Can you work these out from the model? Positions are in its coordinate system, mm. Face numbers are marked on the shaded views. A direction names the side the tool comes from. Give positions to 0.01 mm unless a question says otherwise; leave off trailing zeros. Loops run counter-clockwise (first coordinate to the right, second up) from the corner with the lowest first, then second, coordinate; pieces in that order, holes last.
Autodesk Fusion 360 part; units mm, degrees
sketch "Sketch1" plane through (0, 0, 0) normal (0, 0, 1) x (1, 0, 0)
  line L0 (10, 0) -> (59, 0)
  line L1 (69, 10) -> (69, 170)
  line L2 (59, 180) -> (10, 180)
  line L3 (0, 170) -> (0, 10)
  arc A0 (10, 180) -> (0, 170) centre (10, 170) ccw
  arc A1 (69, 170) -> (59, 180) centre (59, 170) ccw
  arc A2 (59, 0) -> (69, 10) centre (59, 10) ccw
  arc A3 (0, 10) -> (10, 0) centre (10, 10) ccw
  point P0 (69, 0)
  point P1 (0, 180)
  dimension "d1" = 69
  dimension "d2" = 180
  dimension "d3" = 10
  dimension "d4" = 10
  dimension "d5" = 10
sketch "Sketch2" plane through (0, 0, 27) normal (0, 0, 1) x (-1, 0, 0)
  line L0 (-10, 0) -> (-59, 0)
  arc A0 (-59, 0) -> (-69, -10) centre (-59, -10) ccw
sketch "Sketch3" plane through (0, 0, 0) normal (0, 0, 1) x (1, 0, 0)
  line L0 (15, 0) -> (54, 0)
  line L1 (69, 15) -> (69, 180)
  line L2 (54, 195) -> (15, 195)
  line L3 (0, 180) -> (0, 15)
  circle A0 centre (34.5, 110) radius 11
  circle A1 centre (34.5, 85) radius 11
  circle A2 centre (34.5, 128.9) radius 5
  circle A3 centre (34.5, 66.1) radius 5
  circle A4 centre (34.5, 47.2) radius 11
  circle A5 centre (34.5947, 147.7998) radius 11
  circle A6 centre (34.5, 22.2) radius 11
  circle A7 centre (34.4989, 172.7996) radius 11
  arc A8 (15, 195) -> (0, 180) centre (15, 180) ccw
  arc A9 (69, 180) -> (54, 195) centre (54, 180) ccw
  arc A10 (54, 0) -> (69, 15) centre (54, 15) ccw
  arc A11 (0, 15) -> (15, 0) centre (15, 15) ccw
  circle A12 centre (54, 160.2997) radius 4
  point P0 (69, 0)
  dimension "d76" = 22
  dimension "d77" = 22
  dimension "d78" = 18.9
  dimension "d79" = 18.9
  dimension "d80" = 10
  dimension "d81" = 10
  dimension "d82" = 18.9
  dimension "d83" = 18.9
  dimension "d84" = 22
  dimension "d85" = 22
  dimension "d86" = 25
  dimension "d87" = 25
  dimension "d88" = 22
  dimension "d89" = 22
  dimension "d90" = 15
  dimension "d91" = 15
  dimension "d92" = 15
  dimension "d93" = 15
  dimension "d130" = 8
sketch "Sketch4" plane through (0, 0, 27) normal (0, 0, 1) x (-1, 0, 0)
sketch "Sketch5" plane through (0, 0, 0) normal (0, 0, 1) x (1, 0, 0)
extrude "Extrude2" add sketch "Sketch3" along normal blind 27
sketch "Sketch6" plane through (0, 0, 0) normal (0, 0, -1) x (1, 0, 0)
  circle A0 centre (54, -160.2997) radius 4
  circle A1 centre (34.4989, -172.7996) radius 11
  circle A2 centre (34.5, -110) radius 11
  circle A3 centre (34.5947, -147.7998) radius 11
  circle A4 centre (34.5, -85) radius 11
  circle A5 centre (34.5, -66.1) radius 5
  circle A6 centre (34.5, -47.2) radius 11
  circle A7 centre (34.5, -22.2) radius 11
  circle A8 centre (34.5, -128.9) radius 5
  arc A9 (15, 0) -> (0, -15) centre (15, -15) ccw
  line L0 (0, -15) -> (0, -180)
  arc A10 (0, -180) -> (15, -195) centre (15, -180) ccw
  line L1 (15, -195) -> (54, -195)
  arc A11 (54, -195) -> (69, -180) centre (54, -180) ccw
  line L2 (69, -180) -> (69, -15)
  arc A12 (69, -15) -> (54, 0) centre (54, -15) ccw
  line L3 (54, 0) -> (15, 0)
  line L4 (34.5, -85) -> (0, -85)
  line L5 (15, -5) -> (54, -5)
  line L6 (64, -15) -> (64, -180)
  line L7 (54, -190) -> (15, -190)
  line L8 (5, -180) -> (5, -15)
  arc A13 (15, -5) -> (5, -15) centre (15, -15) ccw
  arc A14 (64, -15) -> (54, -5) centre (54, -15) ccw
  arc A15 (5, -180) -> (15, -190) centre (15, -180) ccw
  arc A16 (54, -190) -> (64, -180) centre (54, -180) ccw
  dimension "d162" = 10
  dimension "d163" = 10
  dimension "d164" = 10
  dimension "d165" = 10
extrude "Extrude3" cut sketch "Sketch6" against normal blind 22 contours L5 L6 L7 L8 A13 A14 A15 A16
sketch "Sketch7" plane through (0, 0, 27) normal (0, 0, 1) x (-1, 0, 0)
  circle A0 centre (-54, -160.2997) radius 4
  circle A1 centre (-34.4989, -172.7996) radius 11
  circle A2 centre (-34.5, -110) radius 11
  circle A3 centre (-34.5947, -147.7998) radius 11
  circle A4 centre (-34.5, -85) radius 11
  circle A5 centre (-34.5, -66.1) radius 5
  circle A6 centre (-34.5, -47.2) radius 11
  circle A7 centre (-34.5, -22.2) radius 11
  circle A8 centre (-34.5, -128.9) radius 5
  arc A9 (0, -15) -> (-15, 0) centre (-15, -15) ccw
  line L0 (-15, 0) -> (-54, 0)
  arc A10 (-54, 0) -> (-69, -15) centre (-54, -15) ccw
  line L1 (-69, -15) -> (-69, -180)
  arc A11 (-69, -180) -> (-54, -195) centre (-54, -180) ccw
  line L2 (-54, -195) -> (-15, -195)
  arc A12 (-15, -195) -> (0, -180) centre (-15, -180) ccw
  line L3 (0, -180) -> (0, -15)
sketch "Sketch8" plane through (0, 0, 0) normal (0, 0, -1) x (1, 0, 0)
  line L0 (54, -190) -> (15, -190)
  arc A0 (5, -180) -> (15, -190) centre (15, -180) ccw
  line L1 (5, -180) -> (5, -15)
  arc A1 (15, -5) -> (5, -15) centre (15, -15) ccw
  line L2 (15, -5) -> (54, -5)
  arc A2 (64, -15) -> (54, -5) centre (54, -15) ccw
  line L3 (64, -15) -> (64, -180)
  arc A3 (54, -190) -> (64, -180) centre (54, -180) ccw
  arc A4 (15, 0) -> (0, -15) centre (15, -15) ccw
  line L4 (0, -15) -> (0, -180)
  arc A5 (0, -180) -> (15, -195) centre (15, -180) ccw
  line L5 (15, -195) -> (54, -195)
  arc A6 (54, -195) -> (69, -180) centre (54, -180) ccw
  line L6 (69, -180) -> (69, -15)
  arc A7 (69, -15) -> (54, 0) centre (54, -15) ccw
  line L7 (54, 0) -> (15, 0)
  line L8 (0, -34.7) -> (0, -29.7)
  line L9 (0, -34.7) -> (0, -39.7)
  line L10 (0, -39.7) -> (0, -29.7)
  line L11 (0, -29.7) -> (5, -29.7)
  line L12 (0, -39.7) -> (5, -39.7)
  line L13 (5, -29.7) -> (5, -39.7)
extrude "Extrude4" cut sketch "Sketch8" against normal blind 5 contours L1 L4 L8 L9 L10 L11 L12 L13
sketch "Sketch9" plane through (0, 0, 0) normal (-1, 0, 0) x (0, -1, 0)
  line L0 (-39.7, 0) -> (-39.7, 5)
  line L1 (-39.7, 5) -> (-29.7, 5)
  line L2 (-29.7, 5) -> (-29.7, 0)
  line L3 (-29.7, 0) -> (-15, 0)
  line L4 (-15, 0) -> (-15, 27)
  line L5 (-15, 27) -> (-180, 27)
  line L6 (-180, 27) -> (-180, 0)
  line L7 (-180, 0) -> (-39.7, 0)
  line L8 (-29.7, 0) -> (-29.7, 3)
  line L9 (-31.7, 5) -> (-37.7, 5)
  line L10 (-39.7, 3) -> (-39.7, 0)
  arc A0 (-29.7, 3) -> (-31.7, 5) centre (-31.7, 3) ccw
  arc A1 (-37.7, 5) -> (-39.7, 3) centre (-37.7, 3) ccw
  dimension "d176" = 2
  dimension "d177" = 2
extrude "Extrude5" add sketch "Sketch9" against normal blind 5 contours L0 L1 A1 | L1 L2 A0
sketch "Sketch10" plane through (0, 0, 0) normal (-1, 0, 0) x (0, -1, 0)
  line L0 (-39.7, 0) -> (-39.7, 3)
  arc A0 (-37.7, 5) -> (-39.7, 3) centre (-37.7, 3) ccw
  line L1 (-37.7, 5) -> (-31.7, 5)
  arc A1 (-29.7, 3) -> (-31.7, 5) centre (-31.7, 3) ccw
  line L2 (-29.7, 3) -> (-29.7, 0)
  line L3 (-29.7, 0) -> (-15, 0)
  line L4 (-15, 0) -> (-15, 27)
  line L5 (-15, 27) -> (-180, 27)
  line L6 (-180, 27) -> (-180, 0)
  line L7 (-180, 0) -> (-39.7, 0)
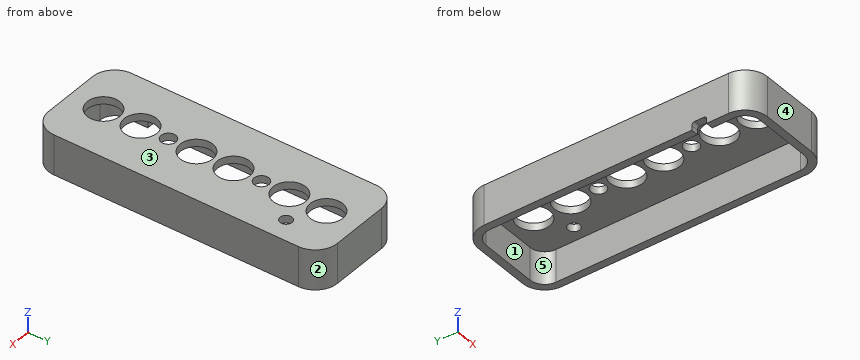
(1) Will these pins go through, and if not, where does the flat tip stop? P1, Ø1, axis at x = 12.5, z = 4, coming from the +Y side; P2, Ø13, axis at x = 34.5, y = 47.2, coming from the -Z side; P3, Ø11.5, axis at x = 34.5, y = 128.9, coming from the +Z side; P4, Ø1.5, axis at x = 3.5, z = 1, coming from the -Y side.
Returned:
P1: stops at y = 194.87
P2: passes through
P3: stops at z = 27
P4: stops at y = 4.54
(2) Thinking about a two-plate mould opening in Y: for the marked faces 1, 2 and 3, which applies, pulls with the +Y half, pulls with the -Y half, needs draft (parallel to the pull), parting line crosses it, or undercut?
Returned:
face 1: undercut
face 2: pulls with the +Y half
face 3: needs draft
(3) Suppose I cut it at A-A on z = 8.75. List the corners of the cut face in (x, y) for me.
Returned:
outline: (0, 15) arc R15 ccw to (15, 0) - (54, 0) arc R15 ccw to (69, 15) - (69, 180) arc R15 ccw to (54, 195) - (15, 195) arc R15 ccw to (0, 180) - close; hole (5, 15) arc R10 ccw to (15, 5) - (54, 5) arc R10 ccw to (64, 15) - (64, 180) arc R10 ccw to (54, 190) - (15, 190) arc R10 ccw to (5, 180) - close
(4) Which directions (+Z, -Z, +X, -X, +Y, -Y) give clear straight access to the entire face, cutting with the end or side of a thin tool? Please do the marked faces 4 and 5.
Returned:
face 4: +Z, -Z, +X, -X, -Y
face 5: -Z
(5) Please list where these lines run through material, in increasing order: probe 1 along X at (y, z) = (22.2, 23.95); probe 2 along X at (y, z) = (14.5, 17.5); probe 3 along Y at (x, z) = (54, 24.55).
Returned:
probe 1: x = 0 to 23.5, 45.5 to 69
probe 2: x = 0.01 to 5.01, 63.99 to 68.99
probe 3: y = 0 to 156.3, 164.3 to 195
(6) Suppose I cut it at B-B on y = 110. List the corners of the cut face in (x, z) for me.
Returned:
outline: (0, 0) - (5, 0) - (5, 22) - (23.5, 22) - (23.5, 27) - (0, 27) - close; (45.5, 22) - (64, 22) - (64, 0) - (69, 0) - (69, 27) - (45.5, 27) - close
(7) Suppose I cut it at D-D on x = 34.5. Give the number of separate pieces and of enclosed holes in the cut face, plus the area to 3 significant figures.
Returned:
separate pieces: 9
enclosed holes: 0
area: 435 mm2
(8) Suppose I cut it at C-C on x = 56. List the corners of the cut face in (y, z) for me.
Returned:
outline: (0.13, 0) - (5.2, 0) - (5.2, 22) - (156.84, 22) - (156.84, 27) - (0.13, 27) - close; (163.76, 22) - (189.8, 22) - (189.8, 0) - (194.87, 0) - (194.87, 27) - (163.76, 27) - close
